Autodesk Inventor part; units mm, degrees
ref_plane "Work Plane1" through (0, 0, -15) normal (0, 0, 1) x (1, 0, 0)
ref_plane "YZ Plane" through (0, 0, 0) normal (1, 0, 0) x (0, 1, 0)
ref_plane "XZ Plane" through (0, 0, 0) normal (0, 1, 0) x (-1, 0, 0)
sketch "Sketch1" plane through (0, 0, 0) normal (0, 0, 1) x (1, 0, 0)
  line L0 (0, 0) -> (25, 0)
  line L1 (25, 0) -> (25, 40)
  line L2 (25, 40) -> (0, 40)
  line L3 (0, 40) -> (0, 0)
  dimension "d1" = 25
  dimension "d2" = 40
  dimension "d3" = 25
extrude "Extrusion1" add sketch "Sketch1" against normal blind 30
sketch "Sketch2" plane through (25, 0, 0) normal (1, 0, 0) x (0, 0, -1)
  line L0 (0, 0) -> (30, 0)
  circle A0 centre (15, 6.56) radius 2.46
extrude "Extrusion2" cut sketch "Sketch2" against normal blind 30
sketch "Sketch3" plane through (0, 0, 0) normal (-1, 0, 0) x (0, 0, 1)
  line L0 (0, 0) -> (-30, 0)
  line L1 (-25.05, 0) -> (-4.95, 0)
  line L2 (-4.95, 0) -> (-4.95, 33.12)
  line L3 (-4.95, 33.12) -> (-25.05, 33.12)
  line L4 (-25.05, 33.12) -> (-25.05, 0)
  dimension "d11" = 20.1
extrude "Extrusion3" cut sketch "Sketch3" against normal blind 20
sketch "Sketch4" plane through (0, 0, 0) normal (0, -1, 0) x (1, 0, 0)
  line L0 (20, -4.95) -> (20, -25.05)
  line L1 (20, -15) -> (25, -15)
  line L2 (25, 0) -> (25, -30)
  line L3 (20, -8.025) -> (25, -8.025)
  line L4 (25, -8.025) -> (25, -21.975)
  line L5 (25, -21.975) -> (20, -21.975)
  line L6 (20, -21.975) -> (20, -8.025)
  line L7 (20, -8.025) -> (25, -21.975) construction
  line L8 (25, -8.025) -> (20, -21.975) construction
  line L9 (25, -12.54) -> (25, -17.46)
  point P0 (0, 0)
  point P1 (22.5, -15)
  dimension "d14" = 13.95
extrude "Extrusion4" add sketch "Sketch4" along normal blind 15
sketch "Sketch5" plane through (20, 0, 0) normal (-1, 0, 0) x (0, 0, 1)
  circle A0 centre (-15, 6.56) radius 2.46
  circle A1 centre (-15, 6.56) radius 4.7025
  circle A2 centre (-15, 6.56) radius 2.46
  circle A3 centre (-15, 6.56) radius 2.46
  point P0 (0, 0)
  dimension "d17" = 9.405
extrude "Extrusion5" cut sketch "Sketch5" against normal blind 2.1
sketch "Sketch6" plane through (25, 0, 0) normal (1, 0, 0) x (0, 0, -1)
  circle A0 centre (15, 6.56) radius 4.7025
  line L0 (15, 6.56) -> (15, 23.56)
  circle A1 centre (15, 23.56) radius 2.46
  point P0 (0, 0)
  dimension "d20" = 17
  dimension "d21" = 4.92
extrude "Extrusion6" cut sketch "Sketch6" against normal blind 10 contours A1
sketch "Sketch7" plane through (20, 0, 0) normal (-1, 0, 0) x (0, 0, 1)
  circle A0 centre (-15, 23.56) radius 2.46
  circle A1 centre (-15, 23.56) radius 4.7025
  point P0 (0, 0)
  dimension "d24" = 9.405
extrude "Extrusion7" cut sketch "Sketch7" against normal blind 2.1
sketch "Sketch9" plane through (25, 0, 0) normal (1, 0, 0) x (0, 0, -1)
  circle A0 centre (15, 6.56) radius 2.46
  circle A1 centre (15, 6.56) radius 2.46
  circle A2 centre (15, 23.56) radius 2.46
  circle A3 centre (15, 23.56) radius 2.46
  line L0 (30, 40) -> (30, 0)
  line L1 (30, 0) -> (30, 40)
  line L2 (30, 40) -> (0, 40)
  line L3 (0, 40) -> (0, 0)
  line L4 (0, 0) -> (8.025, 0)
  line L5 (21.975, 0) -> (21.975, -15)
  line L6 (21.975, -15) -> (8.025, -15)
  line L7 (8.025, -15) -> (8.025, 0)
  line L8 (0, 0) -> (8.025, 0)
  line L9 (21.975, 0) -> (30, 0)
extrude "Extrusion8" add sketch "Sketch9" along normal blind 5
sketch "Sketch10" plane through (0, 40, 0) normal (0, 1, 0) x (1, 0, 0)
  line L0 (0, 30) -> (30, 30)
  line L1 (30, 0) -> (0, 0)
  line L2 (0, 30) -> (30, 30)
  line L3 (30, 30) -> (30, 0)
  line L4 (30, 0) -> (0, 0)
  line L5 (0, 0) -> (0, 30)
extrude "Extrusion9" add sketch "Sketch10" along normal blind 30
sketch "Sketch12" plane through (30, 0, 0) normal (1, 0, 0) x (0, 0, -1)
  circle A0 centre (15, 6.56) radius 2.46
  line L0 (15, 6.56) -> (15, 15.06)
  circle A1 centre (15, 15.06) radius 2.525
  point P0 (0, 0)
  dimension "d31" = 8.5
  dimension "d33" = 5.05
extrude "Extrusion10" cut sketch "Sketch12" against normal blind 30 contours A1
sketch "Sketch14" plane through (0, 0, 0) normal (0, 0, 1) x (1, 0, 0)
  line L0 (30, 70) -> (0, 70)
  line L1 (0, 100) -> (-8, 100)
  line L2 (30, 0) -> (30, 70)
  line L3 (30, 118) -> (30, 70)
  line L4 (30, 105) -> (30, 100)
  line L5 (0, 70) -> (30, 70)
  line L6 (0, 70) -> (0, 100)
  line L7 (30, 122.5) -> (30, 118)
  line L8 (30, 70) -> (30, 145)
  line L9 (-2, 157.5) -> (-8, 160)
  line L10 (-2, 102.5) -> (-8, 100)
  line L11 (4, 130) -> (-2, 102.5)
  line L12 (4, 130) -> (-2, 157.5)
  line L13 (-8, 160) -> (15, 160)
  line L14 (30, 145) -> (15, 160)
  point P0 (0, 0)
  dimension "d47" = 30
extrude "Extrusion12" add sketch "Sketch14" against normal blind 30
sketch "Sketch15" plane through (0, 0, -25.05) normal (-1, 0, 0) x (0, 0, 1)
  line L0 (0, 33.12) -> (20.1, 33.12)
  line L1 (20.1, 33.12) -> (20.1, 0)
  line L2 (0, 33.12) -> (20.1, 33.12)
  line L3 (20.1, 33.12) -> (20.1, 31.1)
  line L4 (20.1, 31.1) -> (0, 31.1)
  line L5 (0, 31.1) -> (0, 33.12)
  point P0 (25.05, 0)
  dimension "d57" = 2.02
extrude "Extrusion13" add sketch "Sketch15" against normal blind 20
sketch "Sketch27" plane through (0, 0, 0) normal (0, 0, 1) x (1, 0, 0)
  point P0 (0, 0)
sketch "Sketch28" plane through (0, 0, 0) normal (0, 0, 1) x (1, 0, 0)
  line L0 (0, 100) -> (-8, 100)
  line L1 (0, 100) -> (-8, 100)
  line L2 (-8, 100) -> (-2, 102.5)
  line L3 (-8, 100) -> (-2, 102.5)
  line L4 (-2, 102.5) -> (4, 130)
  line L5 (-2, 102.5) -> (4, 130)
  line L6 (4, 130) -> (-2, 157.5)
  line L7 (4, 130) -> (-2, 157.5)
  line L8 (-2, 157.5) -> (-8, 160)
  line L9 (-2, 157.5) -> (-8, 160)
  line L10 (-8, 160) -> (15, 160)
  line L11 (-8, 160) -> (15, 160)
  line L12 (15, 160) -> (30, 145)
  line L13 (15, 160) -> (30, 145)
  line L14 (30, 145) -> (30, 93)
  line L15 (30, 0) -> (30, 145)
  line L16 (30, 93) -> (0, 93)
  line L17 (0, 0) -> (0, 100)
  line L18 (0, 93) -> (0, 100)
  dimension "d98" = 52
extrude "Extrusion14" add sketch "Sketch28" along normal blind 30
ref_plane "Work Plane1" through (0, 0, -15) normal (0, 0, 1) x (1, 0, 0)
mirror "Mirror1" about plane through (0, 0, -15) normal (0, 0, 1) of "Extrusion14"
properties part number "55mm_x_90mm"
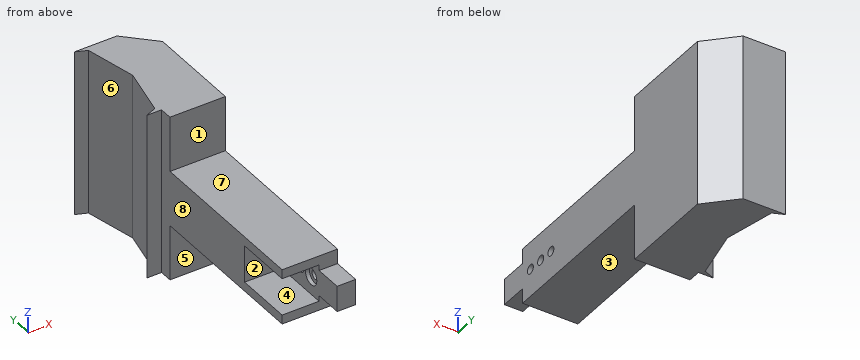
The model under review builds one solid part; all positions refer to its coordinate system, in mm. Face numbers are marked on the shaded views. A direction names the side the tool comes from. Round coordinates to 2 decimals unless told otherwise and drop trailing zeros. Write each loop counter-clockwise with the first axis right and the second up, starting at its lowest first coordinate (ties: lowest second). Pieces come first, ordered by that corner, then holes. Notation, with made-up numbers: (59, 83.5) - (95, 83.5) arc R22 ccw to (95, 89.5) - close; hole circle Ø11 at (38.5, 43). An arc over 180 degrees is marked (long way). Answer as CSV lines item,"result". Start each with the question number.
(1) Draft analysis for pull direction Z (two halves, no side actions). For the marked faces 1, 2 and 3, state which applies: pulls with the +Z half, pulls with the -Z half, needs draft (parallel to the pull), parting line crosses it, or undercut.
(2) We need section C-C on x = 17. State the section outline as (y, z) points, plus the area to 3 significant figures.
(3) To check wall thickness, follow line 1 (Z direction, x = 10, y = 14); line 2 (Y direction, x = 20.8, z = -15) (1 decimal); line 3 (Y direction, x = 25, z = -15) (3 decimals). State the ranges of each line that lie inside material, in increasing order.
(4) We need section D-D on x = -6. State the section outline as (y, z) points, plus the area to 3 significant figures.
(5) We need section B-B on z = -15. Give the number of separate pieces and of enclosed holes in the cut face, plus the area to 3 significant figures.
(6) For pin 1 Ø8 at (y, z) = (70.5, -32) entering from -X; pin 2 Ø9 at (x, z) = (8.5, -5.5) entering from -Y; pin 3 Ø2 at (x, y) = (6.5, 63) entering from -Z, all flat-tipped, find the tip position at first contact; note any pin that passes through.
(7) We need section A-A on y = 15.06. State the section outline as (x, z) points (3 decimals), plus the area to 4 significant figures.
(8) For the marked faces 4, 5, 6, 7 and 8, list the 3-axis set-ups (+Z, -Z, +X, -X, +Y, -Y) from which the entire face can be reached by the end or side of a thin tool; tool diameter is ignored.
Worked answers:
1,face 1,"needs draft"
1,face 2,"undercut"
1,face 3,"pulls with the -Z half"
2,outline,"(0, -30) - (93, -30) - (93, -60) - (158, -60) - (158, 30) - (93, 30) - (93, 0) - (0, 0) - (0, -4.95) - (31.1, -4.95) - (31.1, -25.05) - (0, -25.05) - close"
2,area,"8,010 mm²"
3,line 1,"-30 to -25.05, -4.95 to 0"
3,line 2,"-15 to 1.9, 11.3 to 12.5, 17.6 to 18.9, 28.3 to 154.2"
3,line 3,"-15 to 4.1, 9.02 to 12.535, 17.585 to 21.1, 26.02 to 150"
4,outline,"(100, -60) - (100.83, -60) - (100.83, 30) - (100, 30) - close; (159.17, -60) - (160, -60) - (160, 30) - (159.17, 30) - close"
4,area,"150 mm²"
5,separate pieces,"4"
5,enclosed holes,"0"
5,area,"4,020 mm²"
6,pin 1,"x = 0"
6,pin 2,"y = 0"
6,pin 3,"z = -30"
7,outline,"(0, -30) - (30, -30) - (30, -17.525) - (20, -17.525) - (20, -25.05) - (0, -25.05) - close; (0, -4.95) - (20, -4.95) - (20, -12.475) - (30, -12.475) - (30, 0) - (0, 0) - close"
7,area,"447.5 mm²"
8,face 4,"-X, -Y"
8,face 5,"-Z, +X, -X, -Y"
8,face 6,"+Z, -Z, -X"
8,face 7,"+Z, +X, -X, -Y"
8,face 8,"+Z, -Z, -X, -Y"
